Source: CAD feature listing. Evaluate the final solid. Frame: model axes, mm. A direction names the side the tool comes from. Coordinates: 2 decimals unless noted, no trailing zeros. Write each loop counter-clockwise with the first axis right and the second up, starting at its lowest first coordinate (ties: lowest second). Pieces come first, ordered by that corner, then holes. Notation, with made-up numbers: (9.5, 51) -> (57.5, 51) arc R22 ccw to (57.5, 84) -> close; hole circle Ø1 at (14, -30). An arc over 180 degrees is marked (long way). One line per item, written item: value. Start each with the question number.
1. Section query A-A, the plane y = 13.95. Output: boundary loops of the cut face in (x, z), and give its area (3 significant figures).
2. Access query for faces 4 (the flat face through (-27.5, -9, 20)), 5 (the flat face through (-30, -7.959, 20)), 6 (the flat face through (5, -17, 37)). Directions: +Z, -Z, +X, -X, +Y, -Y. A direction counts if a zero-diameter tool reaches every point of the face in a straight line with its end or side. Return the directions, or none.
3. First-contact query: P1, Ø12, axis at x = -19.5, y = 5, coming from the +Z side; P2, Ø1.5, axis at x = 11, y = 5.5, coming from the +Z side; P3, Ø0.5, axis at x = 3, y = -12, coming from the +Z side; P4, Ø5.5, axis at x = -26, y = -13.5, coming from the +Z side. Flat tips, straight axial feed; report the tip coordinate or a pass-through.
4. Line query: line 1 (Y direction, x = -12.5, z = 15.5); line 2 (Y direction, x = -8, z = 3); line 3 (X direction, y = -14, z = 26.5). Output: solid intervals per line, ascending.
5. Section query D-D, the plane z = 22. Output: boundary loops of the cut face in (x, y), and give its area (3 significant figures).
6. Section query C-C, the plane x = 10.5. Output: boundary loops of the cut face in (y, z).
7. Mould query, pull axis Y, two halves, no side actions, for faces 1 (the flat face through (14.5, 0, 8)), 2 (the flat face through (-32.5, 9, 17)), 3 (the flat face through (24.458, -4.059, 14.297)). Classes: released by +Y, released by -Y, zero draft, split by the parting line, or undercut.
8. Section query B-B, the plane z = 7. State how many separate pieces and enclosed holes the cut face has, and give its area (3 significant figures).
from build123d import *

# Parameters (mm, degrees)
F0_W      = 65
F0_H      = 43
F1_DEPTH  = 2
F2_W      = 65
F2_H      = 43
F2_W_2    = 55
F2_H_2    = 33
F3_DEPTH  = 37
F4_W      = 33
F4_H      = 16
F4_W_2    = 23
F4_H_2    = 13
F5_DEPTH  = 16
F6_R      = 0.9
F7_DEPTH  = 10
F8_W      = 55
F8_H      = 6
F9_DEPTH  = 28
F10_R     = 2.55
F11_DEPTH = 25
F12_R     = 2.75
F13_DEPTH = 25
F15_DEPTH = 29
F16_W     = 31
F16_H     = 6
F17_DEPTH = 1
F18_W     = 16.348152
F18_H     = 34.503732
F19_DEPTH = 5
F20_W     = 24.218268
F20_H     = 6
F21_DEPTH = 8
F22_W     = 6
F22_H     = 16
F23_DEPTH = 5


with BuildPart() as f1:
    # F0 (on Top) → F1 (new body)
    with BuildSketch(Plane.XY):
        Rectangle(F0_W, F0_H)
    extrude(amount=-F1_DEPTH)

    # F2 (on face) → F3 (join)
    with BuildSketch(Plane.XY):
        Rectangle(F2_W, F2_H)
        Rectangle(F2_W_2, F2_H_2, mode=Mode.SUBTRACT)
    extrude(amount=F3_DEPTH)

    # F4 (on face) → F5 (join)
    with BuildSketch(Plane.XY):
        with Locations((3, 0)):
            Rectangle(F4_W, F4_H)
        with Locations((3, 0)):
            Rectangle(F4_W_2, F4_H_2, mode=Mode.SUBTRACT)
    extrude(amount=F5_DEPTH)

    # F6 (on face) → F7 (cut)
    with BuildSketch(Plane.XY.offset(16)):
        with Locations((16.6, 0)):
            Circle(F6_R)
        with Locations((-10.6, 0)):
            Circle(F6_R)
    extrude(amount=-F7_DEPTH, mode=Mode.SUBTRACT)

    # F8 (on face) → F9 (join)
    with BuildSketch(Plane.XY):
        with Locations((0, -13.5)):
            Rectangle(F8_W, F8_H)
        with Locations((0, 13.5)):
            Rectangle(F8_W, F8_H)
    extrude(amount=F9_DEPTH)

    # F10 (on face) → F11 (cut)
    with BuildSketch(Plane(origin=(-32.5, 0, 0), x_dir=(0, -1, 0), z_dir=(-1, 0, 0))):
        with Locations((13.95, 31.65)):
            Circle(F10_R)
        with Locations((-13.95, 31.65)):
            Circle(F10_R)
    extrude(amount=-F11_DEPTH, mode=Mode.SUBTRACT)

    # F12 (on face) → F13 (cut)
    with BuildSketch(Plane.YZ.offset(32.5)):
        with Locations((0, 31.75)):
            Circle(F12_R)
    extrude(amount=-F13_DEPTH, mode=Mode.SUBTRACT)

    # F14 (on face) → F15 (join)
    with BuildSketch(Plane.XY):
        Polygon((21.5, -5.537505), (27.5, -2.537505), (27.5, 2.462495), (21.5, 5.462495), align=None)
    extrude(amount=F15_DEPTH)

    # F16 (on face) → F17 (join)
    with BuildSketch(Plane.XY.offset(28)):
        with Locations((-12, -13.5)):
            Rectangle(F16_W, F16_H)
        with Locations((-12, 13.5)):
            Rectangle(F16_W, F16_H)
    extrude(amount=F17_DEPTH)

    # F18 (on face) → F19 (cut)
    with BuildSketch(Plane(origin=(-32.5, 0, 0), x_dir=(0, -1, 0), z_dir=(-1, 0, 0))):
        with Locations((-0.215107, 19.748134)):
            Rectangle(F18_W, F18_H)
    extrude(amount=-F19_DEPTH, mode=Mode.SUBTRACT)

    # F20 (on face) → F21 (cut)
    with BuildSketch(Plane.XY.offset(29)):
        with Locations((-10.239939, 13.5)):
            Rectangle(F20_W, F20_H)
        with Locations((-10.239939, -13.5)):
            Rectangle(F20_W, F20_H)
    extrude(amount=-F21_DEPTH, mode=Mode.SUBTRACT)

    # F22 (on face) → F23 (cut)
    with BuildSketch(Plane(origin=(-13.5, 0, 0), x_dir=(0, -1, 0), z_dir=(-1, 0, 0))):
        with Locations((0, 8)):
            Rectangle(F22_W, F22_H)
    extrude(amount=-F23_DEPTH, mode=Mode.SUBTRACT)


solid = f1.part
Computed values:
1. outline: (-32.5, -2) -> (32.5, -2) -> (32.5, 37) -> (27.5, 37) -> (27.5, 28) -> (3.5, 28) -> (3.5, 29) -> (1.87, 29) -> (1.87, 21) -> (-22.35, 21) -> (-22.35, 29) -> (-27.5, 29) -> (-27.5, 29.1) -> (-32.5, 29.1) -> close; (-32.5, 34.2) -> (-27.5, 34.2) -> (-27.5, 37) -> (-32.5, 37) -> close
1. area: 1,850 mm²
2. face 4: +Z
2. face 5: +Z, -X
2. face 6: +Z, +X, -X, +Y, -Y
3. P1: stops at z = 21
3. P2: stops at z = 0
3. P3: stops at z = 29
3. P4: stops at z = 37
4. line 1: y = -21.5 to -10.5, -8 to -3, 3 to 8, 10.5 to 21.5
4. line 2: y = -21.5 to -10.5, -8 to -6.5, 6.5 to 8, 10.5 to 21.5
4. line 3: x = -32.5 to -22.35, 1.87 to 32.5
5. outline: (-32.5, -21.5) -> (32.5, -21.5) -> (32.5, 21.5) -> (-32.5, 21.5) -> (-32.5, 8.39) -> (-27.5, 8.39) -> (-27.5, 10.5) -> (-22.35, 10.5) -> (-22.35, 16.5) -> (1.87, 16.5) -> (1.87, 10.5) -> (27.5, 10.5) -> (27.5, 2.46) -> (21.5, 5.46) -> (21.5, -5.54) -> (27.5, -2.54) -> (27.5, -10.5) -> (1.87, -10.5) -> (1.87, -16.5) -> (-22.35, -16.5) -> (-22.35, -10.5) -> (-27.5, -10.5) -> (-27.5, -7.96) -> (-32.5, -7.96) -> close
5. area: 1,320 mm²
6. outline: (-21.5, -2) -> (21.5, -2) -> (21.5, 37) -> (16.5, 37) -> (16.5, 28) -> (10.5, 28) -> (10.5, 0) -> (8, 0) -> (8, 16) -> (6.5, 16) -> (6.5, 0) -> (-6.5, 0) -> (-6.5, 16) -> (-8, 16) -> (-8, 0) -> (-10.5, 0) -> (-10.5, 28) -> (-16.5, 28) -> (-16.5, 37) -> (-21.5, 37) -> close
7. face 1: undercut
7. face 2: zero draft
7. face 3: undercut
8. separate pieces: 2
8. enclosed holes: 1
8. area: 1,800 mm²
